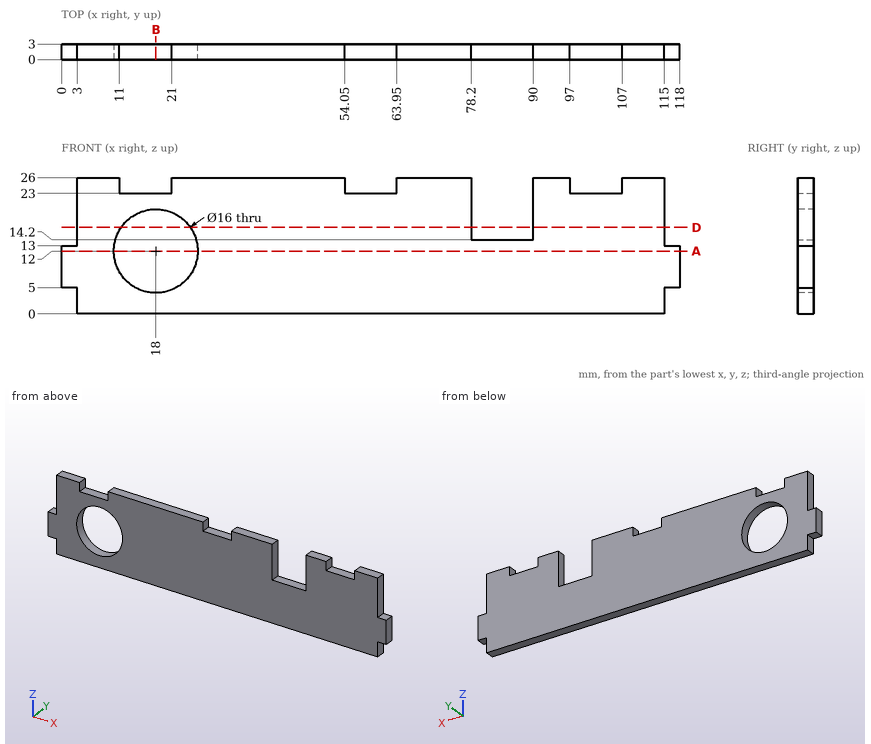
Input: dimensioned drawing with shaded views. Units: mm. Origin: part minimum x, y, z. Give positions to 0.01 mm unless a question says otherwise; leave off trailing zeros. Loops run counter-clockwise (first coordinate to the right, second up) from the corner with the lowest first, then second, coordinate; pieces in that order, holes last. Notation, with made-up numbers: (-14, -36) -> (36, -36) arc R19 cw to (36, -3) -> close; hole circle Ø2 at (-24, 30). An arc over 180 degrees is marked (long way). Use a Markdown table: item, result. Add a question column.
1) First-contact query: pin 1 (0.9 mm diameter, centred on x = 103, y = 1, fed in from +Z); pin 2 (1.5 mm diameter, centred on y = 1, z = 25, fed in from -X); pin 3 (0.9 mm diameter, centred on y = 1.5, z = 24, fed in from +X). Flat tips, straight axial feed; report the tip coordinate or a pass-through.
2) Section query B-B, the plane x = 18. Return the cut outline in (y, z), then the cut area to 3 significant figures.
3) Section query A-A, the plane z = 12. Return the cut outline in (x, y).
4) Section query D-D, the plane z = 16.5. Return the cut outline in (x, y).
5) Line query: line 1 along X through (y, z) = (1.6, 20.5); line 2 along X through (y, z) = (1.15, 12); line 3 along Z through (x, y) = (18, 1.3). Output: solid intervals per line, ascending. Write a range as [from, to].
Numbers:
| question | item | result |
|---|---|---|
| 1 | pin 1 | stops at z = 23 |
| 1 | pin 2 | stops at x = 3 |
| 1 | pin 3 | stops at x = 115 |
| 2 | outline | (0, 0) -> (3, 0) -> (3, 4) -> (0, 4) -> close; (0, 20) -> (3, 20) -> (3, 23) -> (0, 23) -> close |
| 2 | area | 21.0 mm2 |
| 3 | outline | (0, 0) -> (10, 0) -> (10, 3) -> (0, 3) -> close; (26, 0) -> (118, 0) -> (118, 3) -> (26, 3) -> close |
| 4 | outline | (3, 0) -> (11.39, 0) -> (11.39, 3) -> (3, 3) -> close; (24.61, 0) -> (78.2, 0) -> (78.2, 3) -> (24.61, 3) -> close; (90, 0) -> (115, 0) -> (115, 3) -> (90, 3) -> close |
| 5 | line 1 | x = [3, 78.2], [90, 115] |
| 5 | line 2 | x = [0, 10], [26, 118] |
| 5 | line 3 | z = [0, 4], [20, 23] |
